Here's how the part is built. I have some questions about the finished solid (model axes, mm). Face numbers are marked on the shaded views. A direction names the side the tool comes from. Round coordinates to 2 decimals unless told otherwise and drop trailing zeros. Write each loop counter-clockwise with the first axis right and the second up, starting at its lowest first coordinate (ties: lowest second). Pieces come first, ordered by that corner, then holes. Notation, with made-up numbers: M -29.75,-36 L 26.25,-36 A9 ccw 26.25,-29 Z; hole C -17,-8.5 d11. An arc over 180 degrees is marked long. Write item = value, one per line. Start each with the question number.
(1) I want a section at A-A (z = 128.5). List the corners of the cut face in (x, y) for me, and give its area (3 significant figures).
(2) Will these pins go through, and if not, where does the flat tip stop? pin 1 Ø6 at (x, y) = (1, -28.5) entering from +Z; pin 2 Ø2 at (x, z) = (30, 43) entering from +Y; pin 3 Ø8 at (y, z) = (-18.5, 107.5) entering from +X.
(3) If we mould it in two halves opening along Y, with no side actions, what happens to the marked faces 1, 2 and 3? For each: released by +Y, released by -Y, zero draft, split by the parting line, or undercut.
(4) I want a section at C-C (z = 85.5). Give the number of separate pieces and of enclosed holes in the cut face, and give its area (3 significant figures).
(5) On a 3-axis mill with a long thin cutter (end or side, diameter ignored), from which of +Z, -Z, +X, -X, +Y, -Y can I reach the whole of each face in a straight line? I mean the marked faces 4, 5, 6 and 7. Say none if no direction works.
(6) I want a section at B-B (y = 0). List the corners of the cut face in (x, z) for me, and give its area (3 significant figures).
(7) I need wall thicknesses on line 1 along Y through (x, z) = (0, 12.25); line 2 along Z through (x, y) = (5.5, -3.5); line 3 along X through (y, z) = (-14, 22.5). Which ranges of each line are inside material? Lowest first, please.
```python
from build123d import *

# Parameters (mm, degrees)
F0_R      = 26.35
F0_R_2    = 4.75
F1_DEPTH  = 15.3
F10_DEPTH = 50
F11_R     = 10


with BuildPart() as f1:
    # F0 (on Top) → F1 (new body)
    with BuildSketch(Plane.XY):
        Circle(F0_R)
        Circle(F0_R_2, mode=Mode.SUBTRACT)
    extrude(amount=F1_DEPTH)

    # F3 (on offset) → F6 section 0
    with BuildSketch(Plane.XY.offset(15.3)):
        with BuildLine():
            Line((-20.7846096908, -3), (-26.0446251653, -4))
            ThreePointArc((-26.0446251653, -4), (-21.0361208605, -15.8683369999), (-11, -23.944153775))
            Line((-11, -23.944153775), (-8.5, -19.2028643697))
            ThreePointArc((-8.5, -19.2028643697), (-16.7341057315, -12.6873837086), (-20.7846096908, -3))
        make_face()
    # F5 (on offset) → F6 section 1
    with BuildSketch(Plane.XY.offset(90.3)):
        with BuildLine():
            Line((-46.9500885253, -19.917057701), (-49.9299671879, -23.0650899979))
            ThreePointArc((-49.9299671879, -23.0650899979), (-41.5639565173, -36.0199600032), (-29.9302797625, -46.1430206352))
            Line((-29.9302797625, -46.1430206352), (-25.939226182, -43.9107793723))
            ThreePointArc((-25.939226182, -43.9107793723), (-38.3684469263, -33.5985458088), (-46.9500885253, -19.917057701))
        make_face()
    loft()

    # F3 (on offset) → F7 section 0
    with BuildSketch(Plane.XY.offset(15.3)):
        with BuildLine():
            ThreePointArc((11, -23.944153775), (21.0361208605, -15.8683369999), (26.0446251653, -4))
            Line((26.0446251653, -4), (20.7846096908, -3))
            ThreePointArc((20.7846096908, -3), (16.7341057315, -12.6873837086), (8.5, -19.2028643697))
            Line((8.5, -19.2028643697), (11, -23.944153775))
        make_face()
    # F5 (on offset) → F7 section 1
    with BuildSketch(Plane.XY.offset(90.3)):
        with BuildLine():
            ThreePointArc((29.9302797625, -46.1430206352), (41.5639565173, -36.0199600032), (49.9299671879, -23.0650899979))
            Line((49.9299671879, -23.0650899979), (46.9500885253, -19.917057701))
            ThreePointArc((46.9500885253, -19.917057701), (38.3684469263, -33.5985458088), (25.939226182, -43.9107793723))
            Line((25.939226182, -43.9107793723), (29.9302797625, -46.1430206352))
        make_face()
    loft()

    # F3 (on offset) → F8 section 0
    with BuildSketch(Plane.XY.offset(15.3)):
        with BuildLine():
            Line((14.6209088882, 15.0741176618), (10.8002551784, 24.0349118592))
            ThreePointArc((10.8002551784, 24.0349118592), (-1.0259388653, 26.3300199287), (-12.6376925006, 23.1216614511))
            Line((-12.6376925006, 23.1216614511), (-14.6209088882, 15.0741176618))
            ThreePointArc((-14.6209088882, 15.0741176618), (0, 21), (14.6209088882, 15.0741176618))
        make_face()
    # F5 (on offset) → F8 section 1
    with BuildSketch(Plane.XY.offset(90.3)):
        with BuildLine():
            Line((16.5707036778, 48.232891056), (16.4626845195, 52.4783766747))
            ThreePointArc((16.4626845195, 52.4783766747), (0.8932369884, 54.9927461369), (-14.7496566957, 52.9853529512))
            Line((-14.7496566957, 52.9853529512), (-15.3308061409, 48.641200469))
            ThreePointArc((-15.3308061409, 48.641200469), (0.6526987204, 50.9958232052), (16.5707036778, 48.232891056))
        make_face()
    loft()

    # F9 (on offset) → F10 (join)
    with BuildSketch(Plane.XY.offset(90.3)):
        with BuildLine():
            Line((16.5707036778, 48.232891056), (16.4626845195, 52.4783766747))
            ThreePointArc((16.4626845195, 52.4783766747), (0.8932369884, 54.9927461369), (-14.7496566957, 52.9853529512))
            Line((-14.7496566957, 52.9853529512), (-15.3308061409, 48.641200469))
            ThreePointArc((-15.3308061409, 48.641200469), (0.6526987204, 50.9958232052), (16.5707036778, 48.232891056))
        make_face()
        with BuildLine():
            ThreePointArc((-25.939226182, -43.9107793723), (-38.3684469263, -33.5985458088), (-46.9500885253, -19.917057701))
            Line((-46.9500885253, -19.917057701), (-49.9299671879, -23.0650899979))
            ThreePointArc((-49.9299671879, -23.0650899979), (-41.5639565173, -36.0199600032), (-29.9302797625, -46.1430206352))
            Line((-29.9302797625, -46.1430206352), (-25.939226182, -43.9107793723))
        make_face()
        with BuildLine():
            ThreePointArc((46.9500885253, -19.917057701), (38.3684469263, -33.5985458088), (25.939226182, -43.9107793723))
            Line((25.939226182, -43.9107793723), (29.9302797625, -46.1430206352))
            ThreePointArc((29.9302797625, -46.1430206352), (41.5639565173, -36.0199600032), (49.9299671879, -23.0650899979))
            Line((49.9299671879, -23.0650899979), (46.9500885253, -19.917057701))
        make_face()
    extrude(amount=F10_DEPTH)

    # F11
    f11_edges = [f1.edges().sort_by_distance(p)[0] for p in [
        (-41.563957, -36.01996, 90.3),
        (41.563957, -36.01996, 90.3),
        (0.893237, 54.992746, 90.3),
    ]]
    fillet(f11_edges, radius=F11_R)


solid = f1.part
```
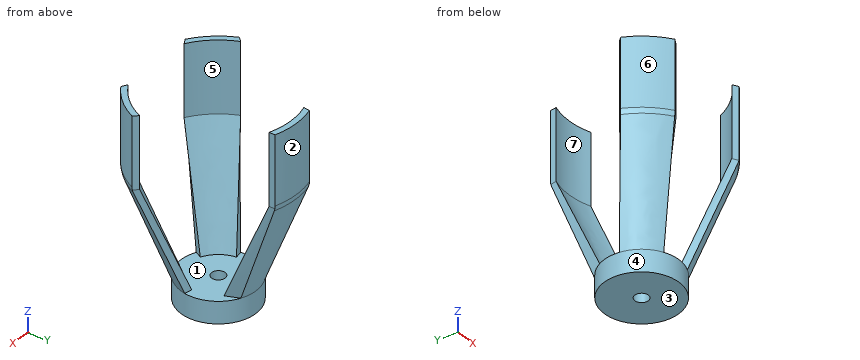
Returned:
q1.outline = M -49.93,-23.07 A55 ccw -29.93,-46.14 L -25.94,-43.91 A51 cw -46.95,-19.92 Z; M -15.33,48.64 A51 cw 16.57,48.23 L 16.46,52.48 A55 ccw -14.75,52.99 Z; M 25.94,-43.91 L 29.93,-46.14 A55 ccw 49.93,-23.07 L 46.95,-19.92 A51 cw Z
q1.area = 382 mm²
q2.pin_1 = 15.3
q2.pin_2 = -9.02
q2.pin_3 = 49.4
q3.face_1 = undercut
q3.face_2 = released by +Y
q3.face_3 = zero draft
q4.separate_pieces = 3
q4.enclosed_holes = 0
q4.area = 385 mm²
q5.face_4 = -Z
q5.face_5 = +Z, +Y
q5.face_6 = +Z, -Z, -X, -Y
q5.face_7 = +Z, -Y
q6.outline = M -26.35,0 L -4.75,0 L -4.75,15.3 L -26.35,15.3 Z; M 4.75,0 L 26.35,0 L 26.35,15.3 L 4.75,15.3 Z
q6.area = 661 mm²
q7.line_1 = -26.35 to -4.75, 4.75 to 26.35
q7.line_2 = 0 to 15.3
q7.line_3 = -25.46 to -19.33, 19.33 to 25.46
